Autodesk Inventor part; units mm, degrees
ref_plane "YZ Plane" through (0, 0, 0) normal (1, 0, 0) x (0, 1, 0)
ref_plane "XZ Plane" through (0, 0, 0) normal (0, 1, 0) x (-1, 0, 0)
ref_plane "XY Plane" through (0, 0, 0) normal (0, 0, 1) x (1, 0, 0)
sketch "Sketch1" plane through (0, 0, 0) normal (0, 0, 1) x (1, 0, 0)
  circle A0 centre (0, 0) radius 17
  circle A1 centre (0, 0) radius 20
  line L0 (-20, 0) -> (20, 0)
  line L1 (0, 0) -> (0, 20.9298)
  line L2 (0, 20.9298) -> (1.5, 20.9298)
  line L3 (1.5, 20.9298) -> (-1.5, 20.9298)
  line L4 (-1.5, 20.9298) -> (-1.5, 15.3128)
  line L5 (-1.5, 15.3128) -> (1.5, 15.3128)
  line L6 (1.5, 15.3128) -> (1.5, 20.9298)
  line L7 (-20, 0) -> (20, 0)
  point P0 (1.5, 19.9437)
  point P1 (1.5, 16.9337)
  point P2 (-1.5, 16.9337)
  point P3 (-1.5, 19.9437)
  dimension "d0" = 34
  dimension "d1" = 40
  dimension "d2" = 1.5
  dimension "d3" = 3
extrude "Extrusion1" add sketch "Sketch1" along normal blind 1.75 contours L0 A1 A0 | A0 L6 A1 L0 | L0 A1 L4 A0
sketch "Sketch2" plane through (0, 0, 1.75) normal (0, 0, 1) x (1, 0, 0)
  arc A0 (-1.5, 19.9437) -> (1.5, 19.9437) centre (0, 0) ccw
  line L0 (0, -20) -> (0, 22)
  line L1 (1.5, 22) -> (6.9, 22)
  line L2 (6.9, 22) -> (6.9, 18.7721)
  line L3 (1.5, 22) -> (1.5, 19.9437)
  arc A1 (-1.5, 19.9437) -> (1.5, 19.9437) centre (0, 0) ccw
  line L4 (-1.5, 22) -> (-6.9, 22)
  line L5 (-6.9, 22) -> (-6.9, 18.7721)
  line L6 (-1.5, 22) -> (-1.5, 19.9437)
  circle A2 centre (-4.2, 18.7721) radius 1
  circle A3 centre (4.2, 18.7721) radius 1
  point P0 (3.7223, 19.6506)
  point P1 (5.0065, 19.3632)
  point P2 (-5.0065, 19.3632)
  point P3 (-3.7223, 19.6506)
  dimension "d7" = 5.4
  dimension "d8" = 2
  dimension "d9" = 2
extrude "Extrusion2" add sketch "Sketch2" against normal blind 1.75 contours A0 A2 L5 L4 L6 | A0 A3 L3 L1 L2
sketch "Sketch3" plane through (0, 0, 0) normal (0, 0, -1) x (-1, 0, 0)
  circle A0 centre (-4.2004, 18.7708) radius 1
  line L0 (0, 22.648) -> (0, 15.9884)
  circle A1 centre (4.2004, 18.7708) radius 1
  point P0 (0, 0)
  dimension "d12" = 2
extrude "Extrusion3" cut sketch "Sketch3" against normal blind 10
fillet "Fillet1" radius 0.6 2 edges at (6.9, 18.7721, 0.875) (-6.9, 18.7721, 0.875)
sketch "Sketch4" plane through (0, 0, 0) normal (0, 0, -1) x (-1, 0, 0)
  circle A0 centre (0, 0) radius 17.5
  line L0 (-17.5, 0) -> (17.5, 0)
  circle A1 centre (0, 0) radius 17
  point P0 (-17, 0)
  point P1 (17, 0)
  dimension "d16" = 35
extrude "Extrusion4" cut sketch "Sketch4" against normal blind 10 contours L0 A1 A0 picked at (-7.3917, 15.5534)
sketch "Sketch5" plane through (17, 0, 0) normal (0, 1, 0) x (1, 0, 0)
  line L0 (0.5, -1.75) -> (0, -1.75)
  line L1 (0, 0) -> (0.5, 0)
  line L2 (0.5, -1.75) -> (0, -1.75)
  line L3 (0, -1.75) -> (0, 0)
  line L4 (0, 0) -> (0.5, 0)
  line L5 (0.5, 0) -> (0.5, -1.75)
  point P0 (-17, 0)
  point P1 (0, -1.75)
extrude "Extrusion5" add sketch "Sketch5" along normal blind 5
fillet "Fillet2" radius 2 1 edges at (17, 4.1533, 0.875)
sketch "Sketch6" plane through (17, 0, 0) normal (-1, 0, 0) x (0, 0, 1)
  point P0 (0, 0)
mirror "Mirror1" about plane through (0, 0, 0) normal (1, 0, 0) of "Extrusion5"
fillet "Fillet3" radius 2 1 edges at (-17, 4.1533, 0.875)
properties part number "cockring"
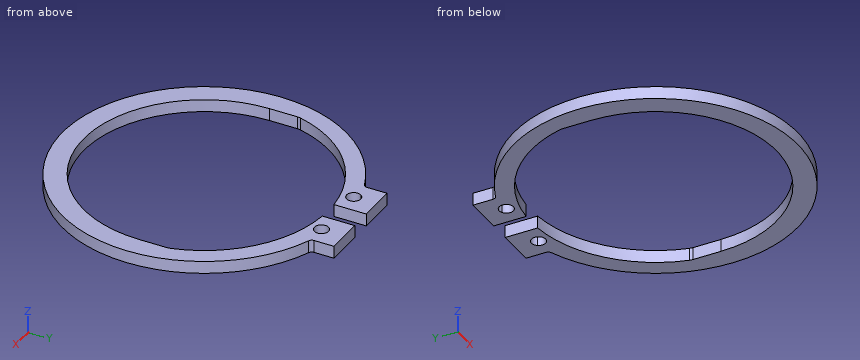
Read the model definition and answer for the solid it produces. Units are mm, in the model's axes. Give positions to 0.01 mm unless a question says otherwise; leave off trailing zeros. Write each loop counter-clockwise with the first axis right and the second up, starting at its lowest first coordinate (ties: lowest second). Pieces come first, ordered by that corner, then holes. Notation, with made-up numbers: (71, 88.5) -> (121, 88.5) arc R27 ccw to (121, 118.5) -> close; hole circle Ø8 at (-39, 84.5). An arc over 180 degrees is marked (long way). Answer as a JSON object with one key per item and string values. Group by question number.
1) Consider L1, parallel to Y at x = -6, z = 0.9; L2, parallel to Y at x = 12, z = 0.4; L3, parallel to X at y = 7.5, z = 1.15. Determine where each line is inside the solid, lowest interval first. Write a range as from..to.
2) Each of these flat-tipped pins is pushed along its axis until it touches: P1, Ø0.5, axis at y = 20.5, z = 1.5, coming from the +X side; P2, Ø0.5, axis at y = 1, z = 1, coming from the -X side; P3, Ø0.5, axis at y = 20, z = 0.5, coming from the -X side; P4, Ø3, axis at x = 15.5, y = 17, coming from the -Z side. Where does it stop, or does it pass through?
3) Find section D-D (x = 0). Write down the section's boundary in (y, z), and give its area (3 significant figures).
4) Find section B-B (y = -4.5). Write down the section's boundary in (x, z).
5) Find section A-A (x = 14.5). Write down the section's boundary in (y, z).
6) Find section C-C (z = 1.3). Count the separate pieces of the cut face and the enclosed holes in it, and give its area (3 significant figures).
Values follow:
{
 "1": {"L1": "y = -19.08..-15.91, 16.44..22", "L2": "y = -16..-12.04, 12.74..16", "L3": "x = -18.54..-15.81, 15.81..18.54"},
 "2": {"P1": "stops at x = 6.9", "P2": "stops at x = -19.99", "P3": "stops at x = -6.9", "P4": "passes through"},
 "3": {"outline": "(-20, 0) -> (-17, 0) -> (-17, 1.75) -> (-20, 1.75) -> close", "area": "5.25 mm2"},
 "4": {"outline": "(-19.49, 0) -> (-16.39, 0) -> (-16.39, 1.75) -> (-19.49, 1.75) -> close; (16.39, 0) -> (19.49, 0) -> (19.49, 1.75) -> (16.39, 1.75) -> close"},
 "5": {"outline": "(-13.77, 0) -> (-8.87, 0) -> (-8.87, 1.75) -> (-13.77, 1.75) -> close; (9.8, 0) -> (13.77, 0) -> (13.77, 1.75) -> (9.8, 1.75) -> close"},
 "6": {"separate pieces": "1", "enclosed holes": "2", "area": "338 mm2"}
}
